Here's the drawing with two shaded views (mm, measured from the low corner). I have some questions. Round coordinates to 2 decimals unless told otherwise and drop trailing zeros. Write each loop counter-clockwise with the first axis right and the second up, starting at its lowest first coordinate (ties: lowest second). Pieces come first, ordered by that corner, then holes. Notation, with made-up numbers: M 81,57 L 133,57 A35 ccw 133,96 Z; hole C -21.5,82 d10. An arc over 180 degrees is marked long. Answer as a JSON object with one key per item and string values. Group by question number.
1) I'm going to push a flat-ended pin straight in: pin 1 Ø4 at (x, z) = (22.5, 11.5) entering from -Y. Where does the tip first touch, or does it pass through?
2) Suppose I cut it at A-A, the plane x = 7.5. Write out the boundary of the cut face in (y, z).
3) Suppose I cut it at D-D, the plane x = 42. Write out the boundary of the cut face in (y, z), and give its area (3 significant figures).
4) Suppose I cut it at C-C, the plane y = 0.85. Write out the boundary of the cut face in (x, z).
5) Please list where these lines run through material, in increasing order: L1, parallel to Z at x = 42.5, y = 0.5; L2, parallel to X at y = 1.15, z = 6.5; L3, parallel to Z at x = 43, y = 1.55. Write a range as [from, to].
6) Suppose I cut it at B-B, the plane z = 7.5. Write out the boundary of the cut face in (x, y), and give its area (3 significant figures).
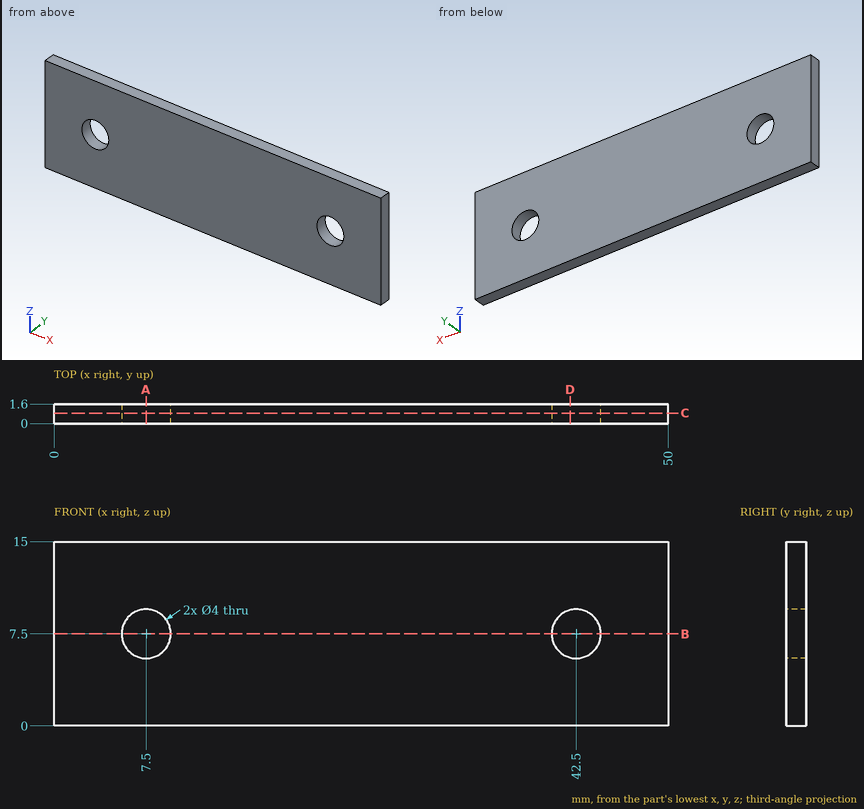
Results:
{
 "1": {"pin 1": "y = 0"},
 "2": {"outline": "M 0,0 L 1.6,0 L 1.6,5.5 L 0,5.5 Z; M 0,9.5 L 1.6,9.5 L 1.6,15 L 0,15 Z"},
 "3": {"outline": "M 0,0 L 1.6,0 L 1.6,5.56 L 0,5.56 Z; M 0,9.44 L 1.6,9.44 L 1.6,15 L 0,15 Z", "area": "17.8 mm^2"},
 "4": {"outline": "M 0,0 L 50,0 L 50,15 L 0,15 Z; hole C 7.5,7.5 d4; hole C 42.5,7.5 d4"},
 "5": {"L1": "[0, 5.5], [9.5, 15]", "L2": "[0, 5.77], [9.23, 40.77], [44.23, 50]", "L3": "[0, 5.56], [9.44, 15]"},
 "6": {"outline": "M 0,0 L 5.5,0 L 5.5,1.6 L 0,1.6 Z; M 9.5,0 L 40.5,0 L 40.5,1.6 L 9.5,1.6 Z; M 44.5,0 L 50,0 L 50,1.6 L 44.5,1.6 Z", "area": "67.2 mm^2"}
}
